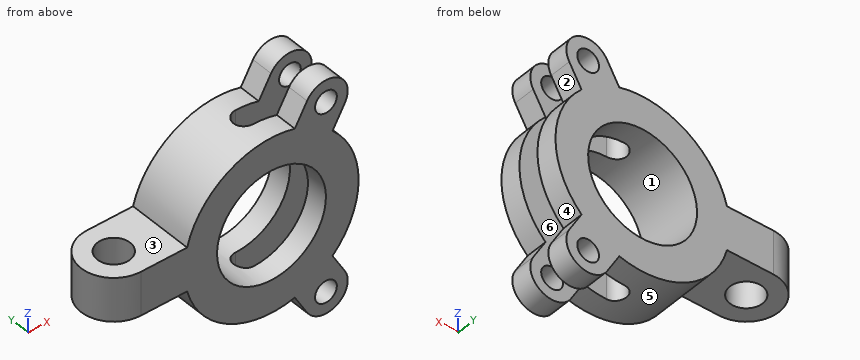
```python
from build123d import *

# Parameters (mm, degrees)
SKETCH1_R               = 40
SKETCH1_R_2             = 25
BOSS_EXTRUDE1_DEPTH     = 15
CUT_EXTRUDE1_DEPTH      = 59.523499554
CUT_EXTRUDE1_DEPTH_BACK = 59.523499554
SKETCH2_R               = 5
SKETCH2_W               = 40
SKETCH2_H               = 10
BOSS_EXTRUDE2_START     = 15
SKETCH3_R               = 5
BOSS_EXTRUDE2_DEPTH     = 10
MIRROR2_START           = 15
MIRROR2_COPY_1_SKETCH_R = 5
MIRROR2_COPY_1_DEPTH    = 10
BOSS_EXTRUDE4_DEPTH     = 10


with BuildPart() as part:
    # Sketch1 → Boss-Extrude1 (new, symmetric)
    with BuildSketch(Plane(origin=(0, 0, 0), x_dir=(1, 0, 0), z_dir=(0, 1, 0))):
        with Locations(Location((0, 0, 0), (0, 0, 270))):
            Circle(SKETCH1_R)
        with Locations(Location((0, 0, 0), (0, 0, 270))):
            Circle(SKETCH1_R_2, mode=Mode.SUBTRACT)
    extrude(amount=BOSS_EXTRUDE1_DEPTH, both=True)

    # Sketch2 → Cut-Extrude1 (cut, two sides: drawn at the far end of the back side and taken through both)
    with BuildSketch(Plane.XY.offset(-CUT_EXTRUDE1_DEPTH_BACK)):
        Circle(SKETCH2_R)
        with Locations((20, 0)):
            Rectangle(SKETCH2_W, SKETCH2_H)
    extrude(amount=CUT_EXTRUDE1_DEPTH + CUT_EXTRUDE1_DEPTH_BACK, mode=Mode.SUBTRACT)

    # Sketch3 → Boss-Extrude2 (add)
    with BuildSketch(Plane(origin=(0, 0, 0), x_dir=(1, 0, 0), z_dir=(0, 1, 0)).offset(BOSS_EXTRUDE2_START)):
        with BuildLine():
            Line((16.339745962, -48.301270189), (10.704662693, -38.541019662))
            ThreePointArc((10.704662693, -38.541019662), (20, -34.641016151), (28.025170769, -28.541019662))
            Line((28.025170769, -28.541019662), (33.660254038, -38.301270189))
            ThreePointArc((33.660254038, -38.301270189), (30, -51.961524227), (16.339745962, -48.301270189))
        make_face()
        with Locations(Location((25, -43.301270189, 0), (0, 0, 270))):
            Circle(SKETCH3_R, mode=Mode.SUBTRACT)
    boss_extrude2 = extrude(amount=-BOSS_EXTRUDE2_DEPTH)

    # Mirror1: Boss-Extrude2 across plane
    add(boss_extrude2.mirror(Plane.XY))

    # Mirror2: Boss-Extrude2 across plane
    add(boss_extrude2.mirror(Plane.ZX))

    # Mirror2 copy 1 sketch → Mirror2 copy 1 (add)
    with BuildSketch(Plane.XZ.offset(MIRROR2_START)):
        with BuildLine():
            Line((16.339745962, -48.301270189), (10.704662693, -38.541019662))
            ThreePointArc((10.704662693, -38.541019662), (20, -34.641016151), (28.025170769, -28.541019662))
            Line((28.025170769, -28.541019662), (33.660254038, -38.301270189))
            ThreePointArc((33.660254038, -38.301270189), (30, -51.961524227), (16.339745962, -48.301270189))
        make_face()
        with Locations(Location((25, -43.301270189, 0), (0, 0, 270))):
            Circle(MIRROR2_COPY_1_SKETCH_R, mode=Mode.SUBTRACT)
    extrude(amount=-MIRROR2_COPY_1_DEPTH)

    # Sketch4 → Boss-Extrude4 (add, symmetric)
    with BuildSketch(Plane.XY):
        with BuildLine():
            ThreePointArc((-60, -15), (-49.393398282, -10.606601718), (-45, 0))
            Line((-45, 0), (-52.5, 0))
            ThreePointArc((-52.5, 0), (-60, -7.5), (-67.5, 0))
            Line((-67.5, 0), (-75, 0))
            ThreePointArc((-75, 0), (-70.606601718, -10.606601718), (-60, -15))
        make_face()
        with BuildLine():
            Line((-52.5, 0), (-45, 0))
            ThreePointArc((-45, 0), (-49.393398282, 10.606601718), (-60, 15))
            ThreePointArc((-60, 15), (-70.606601718, 10.606601718), (-75, 0))
            Line((-75, 0), (-67.5, 0))
            ThreePointArc((-67.5, 0), (-60, 7.5), (-52.5, 0))
        make_face()
        with BuildLine():
            ThreePointArc((-60, 15), (-49.393398282, 10.606601718), (-45, 0))
            Line((-45, 0), (-25, 0))
            Line((-25, 0), (-25, 15))
            Line((-25, 15), (-60, 15))
        make_face()
        with BuildLine():
            Line((-25, 0), (-45, 0))
            ThreePointArc((-45, 0), (-49.393398282, -10.606601718), (-60, -15))
            Line((-60, -15), (-25, -15))
            Line((-25, -15), (-25, 0))
        make_face()
    extrude(amount=BOSS_EXTRUDE4_DEPTH, both=True)


solid = part.part
```
Here's how the part is built. I have some questions about the finished solid (model axes, mm). Face numbers are marked on the shaded views. A direction names the side the tool comes from. Coordinates: 2 decimals unless noted, no trailing zeros. Loops run counter-clockwise (first coordinate to the right, second up) from the corner with the lowest first, then second, coordinate; pieces in that order, holes last. Notation, with made-up numbers: M 49,50.25 L 93,50.25 A23 cw 93,81.25 Z; hole C 80.5,51.25 d8. An arc over 180 degrees is marked long. One line per item, written item: value.
1. Will these pins go through, and if not, where does the flat tip stop? pin 1 Ø12 at (x, y) = (-16, -1) entering from -Z; pin 2 Ø5 at (y, z) = (7.5, 38) entering from +X; pin 3 Ø9 at (x, y) = (-66, 0.5) entering from +Z.
Geometry says:
pin 1: stops at z = -38.73
pin 2: stops at x = 34.6
pin 3: stops at z = 10
2. Imagine slicing it at A-A (z = 0). List the corners of the cut face in (x, y) for me, and give its area (3 significant figures).
Geometry says:
outline: M -60,-15 L -25,-15 L -25,15 L -60,15 A15 ccw Z; M 25,-15 L 40,-15 L 40,-5 L 25,-5 Z; M 25,5 L 40,5 L 40,15 L 25,15 Z; hole C -60,0 d15
area: 1,530 mm2
3. On a 3-axis mill with a long thin cutter (end or side, diameter ignored), from which of +Z, -Z, +X, -X, +Y, -Y can I reach the whole of each face in a straight line? I mean the marked faces 1, 2 and 3. Say none if no direction works.
Geometry says:
face 1: +Y, -Y
face 2: +X, +Y, -Y
face 3: +Z, -X, +Y, -Y
4. Imagine slicing it at B-B (y = 2.5). List the corners of the cut face in (x, z) for me, and give its area (3 significant figures).
Geometry says:
outline: M -74.79,-10 L -67.07,-10 L -67.07,10 L -74.79,10 Z; M -52.93,-10 L -38.73,-10 A40 ccw -4.33,-39.76 L -4.33,-24.62 A25 cw -4.33,24.62 L -4.33,39.76 A40 ccw -38.73,10 L -52.93,10 Z
area: 1,820 mm2
5. Imagine slicing it at D-D (x = 3.5). List the corners of the cut face in (y, z) for me.
Geometry says:
outline: M -15,-39.85 L -5,-39.85 L -5,-24.75 L -15,-24.75 Z; M -15,24.75 L -5,24.75 L -5,39.85 L -15,39.85 Z; M 5,-39.85 L 15,-39.85 L 15,-24.75 L 5,-24.75 Z; M 5,24.75 L 15,24.75 L 15,39.85 L 5,39.85 Z
6. Imagine slicing it at C-C (z = -46). List the corners of the cut face in (x, y) for me.
Geometry says:
outline: M 15.01,-15 L 20.79,-15 L 20.79,-5 L 15.01,-5 Z; M 15.01,5 L 20.79,5 L 20.79,15 L 15.01,15 Z; M 29.21,-15 L 34.63,-15 L 34.63,-5 L 29.21,-5 Z; M 29.21,5 L 34.63,5 L 34.63,15 L 29.21,15 Z
7. Thinking about a two-plate mould opening in X: for the marked faces 4, 5 and 6, which applies, +X half, -X half, draft (parallel to the pull), parting line (faces both ways), or undercut?
Geometry says:
face 4: +X half
face 5: undercut
face 6: draft
8. Please list where these lines run through material, in increasing order: probe 1 along Y at (x, z) = (28, -15.5); probe 2 along Z at (x, y) = (33, -10); probe 3 along Z at (x, y) = (-50, 11).
Geometry says:
probe 1: y = -15 to -5, 5 to 15
probe 2: z = -49.3 to -37.16, -22.61 to 22.61, 37.16 to 49.3
probe 3: z = -10 to 10
